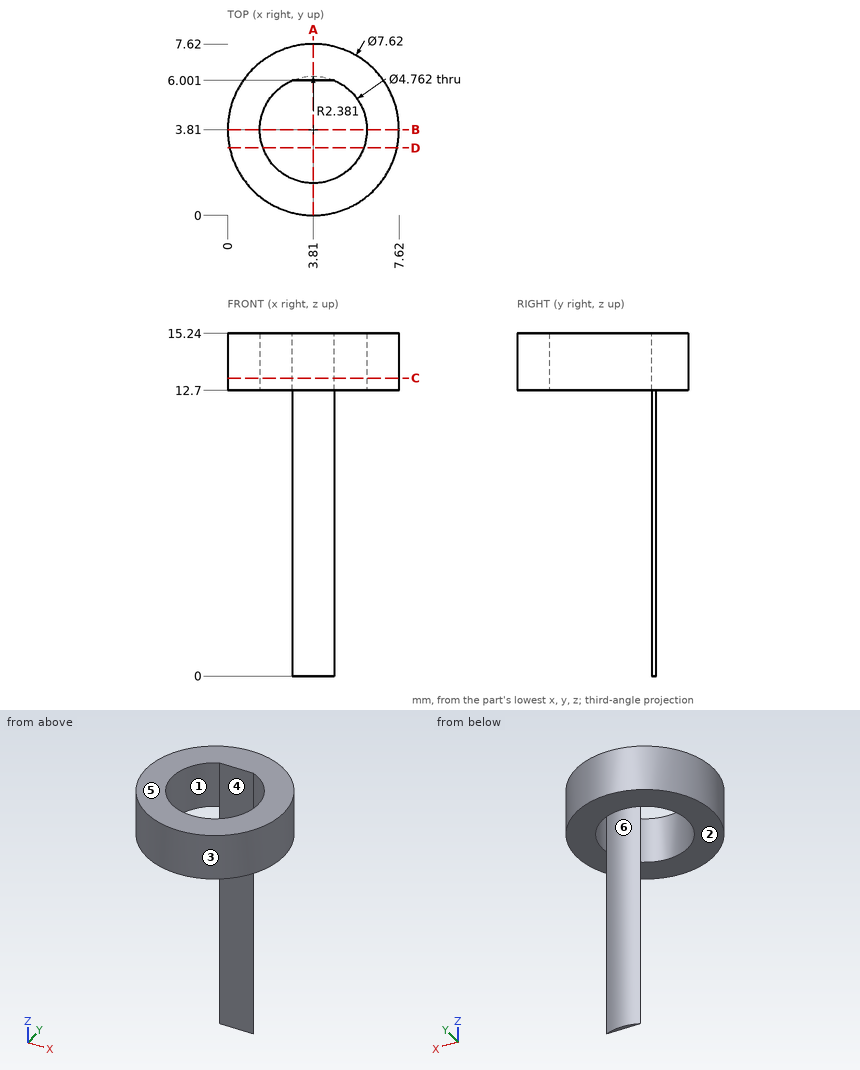
Source: three-view drawing plus pictorial views. Frame: mm from the lowest corner of the part. A direction names the side the tool comes from. Coordinates: 2 decimals unless noted, no trailing zeros. Order: outer loops, then holes, each group sorted by start corner. A loop starts at its lowest first (then second) coordinate and runs counter-clockwise, first axis right, second up.
Item 1: Cut plane D-D (y = 3). Return loops of the section in (x, z).
Output values:
outline: (0.09, 12.7) - (1.57, 12.7) - (1.57, 15.24) - (0.09, 15.24) - close; (6.05, 12.7) - (7.53, 12.7) - (7.53, 15.24) - (6.05, 15.24) - close
Item 2: Set-up query: the marked faces 4, 5 and 6. Return all of +Z, -Z, +X, -X, +Y, -Y with unobstructed straight access to the full face (end or side cutting, diameter ignored); none if empty.
Output values:
face 4: +Z, -Z
face 5: +Z, +X, -X, +Y, -Y
face 6: -Z, +Y
Item 3: Material intervals for line 1 (Y direction, x = 3.81, z = 14); line 2 (Z direction, x = 7, y = 5); line 3 (X direction, y = 4.5, z = 13.25), sorted ascending.
Output values:
line 1: y = 0 to 1.43, 6 to 7.62
line 2: z = 12.7 to 15.24
line 3: x = 0.06 to 1.53, 6.09 to 7.56
Item 4: Pull-direction query (Y, two-part tool) for the marked faces 1, 2 and 3; classes: pulls with the +Y half, pulls with the -Y half, needs draft (parallel to the pull), parting line crosses it, or undercut.
Output values:
face 1: undercut
face 2: needs draft
face 3: parting line crosses it
Item 5: Cut plane B-B (y = 3.81). Return loops of the section in (x, z).
Output values:
outline: (0, 12.7) - (1.43, 12.7) - (1.43, 15.24) - (0, 15.24) - close; (6.19, 12.7) - (7.62, 12.7) - (7.62, 15.24) - (6.19, 15.24) - close
Item 6: Cut plane C-C (z = 13.25). Return loops of the section in (x, y).
Output values:
outline: circle Ø7.62 at (3.81, 3.81); hole (2.88, 6) arc R2.38 ccw (long way) to (4.74, 6) - close
Item 7: First-contact query: P1, Ø2, axis at x = 4, z = 10.5, coming from the -Y side. Flat tip, straight axial feed; report the tip coordinate or a pass-through.
Output values:
P1: stops at y = 6
Item 8: Cut plane A-A (x = 3.81). Return loops of the section in (y, z).
Output values:
outline: (0, 12.7) - (1.43, 12.7) - (1.43, 15.24) - (0, 15.24) - close; (6, 0) - (6.19, 0) - (6.19, 12.7) - (7.62, 12.7) - (7.62, 15.24) - (6, 15.24) - close
